For this review, take the finished solid that the model builds, in its own axes (mm). Face numbers are marked on the shaded views. A direction names the side the tool comes from. Round coordinates to 2 decimals unless told otherwise and drop trailing zeros. Order: outer loops, then holes, each group sorted by start corner. A loop starts at its lowest first (then second) coordinate and runs counter-clockwise, first axis right, second up. Notation, with made-up numbers: (58, 12.5) -> (104, 12.5) arc R14 cw to (104, 17.5) -> close; hole circle Ø2 at (40.5, 61). An arc over 180 degrees is marked (long way). Use a Markdown table: item, result. Add a question column.
1) Clearance check with flat-ended pins moving along their axes: P1, Ø1.5, axis at x = -63.5, z = -161.5, coming from the -Y side; P2, Ø10, axis at x = 65.5, z = -95.5, coming from the +Y side; P3, Ø6, axis at x = 101, y = 11, coming from the +Z side. State where each tip first meets the part, or that it passes through.
2) Machinability: for the marked faces 1, 2 and 3, which of the approach directions +Z, -Z, +X, -X, +Y, -Y give a long, thin tool a straight path to every point of the face, cutting with its end or side? Answer none if there is none.
3) Consider section A-A (x = 235). State the section outline as (y, z) points.
4) Draft analysis for pull direction Y (two halves, no side actions). For the marked faces 4, 5 and 6, state which applies: pulls with the +Y half, pulls with the -Y half, needs draft (parallel to the pull), parting line crosses it, or undercut.
5) Wall thickness on line 1 along Z through (x, y) = (-74.5, 6); line 2 along Z through (x, y) = (-70, 0); line 3 along X through (y, z) = (-265, 0): over which ranges is each line inside the solid? List them lowest first. Write a range as [from, to].
6) Consider section B-B (x = 353.5). State the section outline as (y, z) points, plus the area to 3 significant figures.
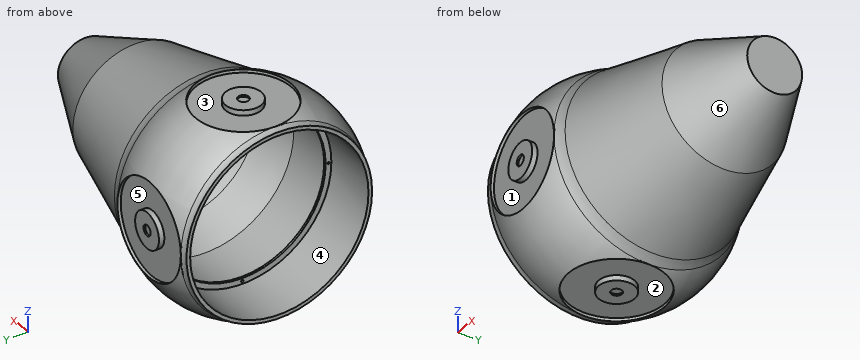
```python
from build123d import *

# Parameters (mm, degrees)
ESCALA1_SCALE               = 0.2
PADR_OCIRCULAR1_COUNT       = 4
FURO_COM_FOLGA_DE_M61_D     = 6.6
FURO_COM_FOLGA_DE_M61_DEPTH = 15.999481013
FURO_COM_FOLGA_DE_M61_TIP   = 1.982840043


with BuildPart() as part:
    # Esboço1 → Revolução1 (revolve)
    with BuildSketch(Plane.XY, mode=Mode.PRIVATE) as revolu_o1_sk:
        with BuildLine():
            Line((3317.399667889, 0), (3317.399667889, 383.5))
            Line((3317.399667889, 383.5), (2265.399667889, 873))
            Line((2265.399667889, 873), (813.399667889, 1260))
            ThreePointArc((813.399667889, 1260), (737.813781205, 1284.220696189), (665, 1315.812176946))
            ThreePointArc((665, 1315.812176946), (0, 1471.161405015), (-665, 1315.812176946))
            ThreePointArc((-665, 1315.812176946), (-708.110967822, 1300.356342101), (-753.607594937, 1295.112746158))
            Line((-753.607594937, 1295.112746158), (-753.607594937, 1244.476357536))
            Line((-753.607594937, 1244.476357536), (25.002405063, 1244.476357536))
            Line((25.002405063, 1244.476357536), (25.002405063, 1164.476357536))
            Line((25.002405063, 1164.476357536), (55.002405063, 1164.476357536))
            Line((55.002405063, 1164.476357536), (55.002405063, 1244.476357536))
            Line((55.002405063, 1244.476357536), (813.399667889, 1244.476357536))
            Line((813.399667889, 1244.476357536), (1370.201096416, 1096.072671007))
            Line((1370.201096416, 1096.072671007), (2260.264870662, 858.844929525))
            Line((2260.264870662, 858.844929525), (3302.399667889, 373.935249636))
            Line((3302.399667889, 373.935249636), (3302.399667889, 0))
            Line((3302.399667889, 0), (3317.399667889, 0))
        make_face()
    revolve(revolu_o1_sk.sketch.rotate(Axis((-14.7457766, 0, 0), (1, 0, 0)), 180), axis=Axis((-14.7457766, 0, 0), (1, 0, 0)))


with BuildPart() as part_1:
    # Escala1: scaled about (0, 0, 0)
    add(part.part.scale(ESCALA1_SCALE))

    # Esboço2 → Corte-Revolução9 (revolve, cut)
    with BuildSketch(Plane.XY, mode=Mode.PRIVATE) as corte_revolu_o9_sk:
        Polygon((15, 268.895271507), (15, 263.895271507), (0, 263.895271507), (0, 311.146389703), (133, 311.146389703), (133, 253.895271507), (50, 253.895271507), (50, 268.895271507), align=None)
    corte_revolu_o9 = revolve(corte_revolu_o9_sk.sketch.rotate(Axis((0, -141.14012245, 0), (0, 1, 0)), 90), axis=Axis((0, -141.14012245, 0), (0, 1, 0)), mode=Mode.SUBTRACT)

    # PadrãoCircular1: Corte-Revolução9 ×4 about axis
    padr_ocircular1_axis = Axis((0, 0, 0), (1, 0, 0))
    for i in range(1, PADR_OCIRCULAR1_COUNT):
        add(corte_revolu_o9.rotate(padr_ocircular1_axis, i * 360 / PADR_OCIRCULAR1_COUNT), mode=Mode.SUBTRACT)

    # Furo com folga de M61
    with Locations(Plane(origin=(11.000481013, 0, 0), x_dir=(0, 0, -1), z_dir=(1, 0, 0))):
        with Locations((0, 240.895271507), (240.895271507, 0), (0, -240.895271507), (-240.895271507, 0), (0, 0)):
            Hole(FURO_COM_FOLGA_DE_M61_D / 2, depth=FURO_COM_FOLGA_DE_M61_DEPTH)
            with Locations((0, 0, -(FURO_COM_FOLGA_DE_M61_DEPTH + FURO_COM_FOLGA_DE_M61_TIP / 2))):  # 118° drill point
                Cone(0, FURO_COM_FOLGA_DE_M61_D / 2, FURO_COM_FOLGA_DE_M61_TIP, mode=Mode.SUBTRACT)


solid = part_1.part
```
Results list:
| question | item | result |
|---|---|---|
| 1 | P1 | y = -238.32 |
| 1 | P2 | y = 253.9 |
| 1 | P3 | z = 253.9 |
| 2 | face 1 | -Y |
| 2 | face 2 | -Z |
| 2 | face 3 | +Z |
| 3 | outline | circle Ø465.45 at (0, 0); hole circle Ø459.24 at (0, 0) |
| 4 | face 4 | undercut |
| 4 | face 5 | pulls with the +Y half |
| 4 | face 6 | parting line crosses it |
| 5 | line 1 | [-253.9, -248.82], [248.82, 253.9] |
| 5 | line 2 | [-253.9, -248.9], [248.9, 253.9] |
| 5 | line 3 | [-50, -15], [15, 50] |
| 6 | outline | circle Ø402.28 at (0, 0); hole circle Ø396.07 at (0, 0) |
| 6 | area | 3,890 mm2 |
